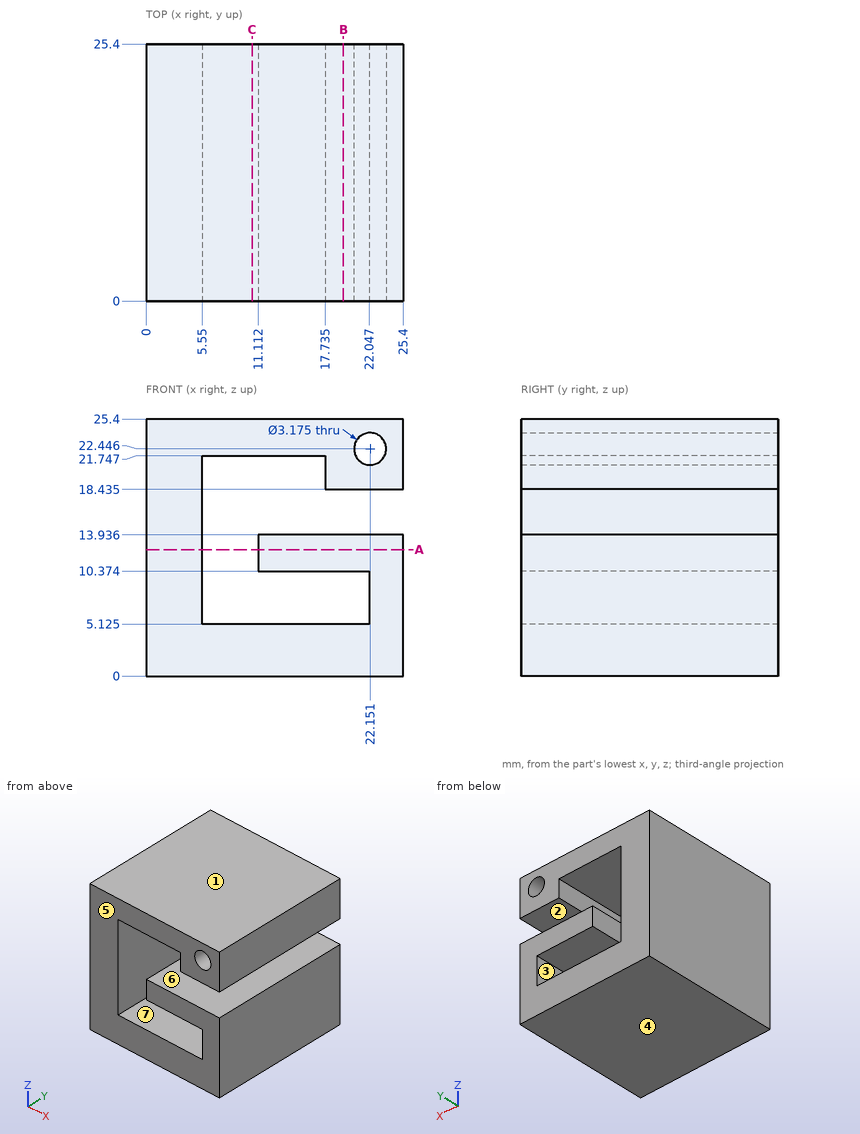
Source: three-view drawing plus pictorial views. Frame: mm from the lowest corner of the part. A direction names the side the tool comes from. Round coordinates to 2 decimals unless told otherwise and drop trailing zeros. Loops run counter-clockwise (first coordinate to the right, second up) from the corner with the lowest first, then second, coordinate; pieces in that order, holes last. Notation, with made-up numbers: (-11.5, 57) -> (28.5, 57) arc R30 ccw to (28.5, 81) -> close; hole circle Ø11 at (-24.75, 4.5). An arc over 180 degrees is marked (long way). Use one line per item in the form item = value.
Item 1: Material intervals for probe 1 along Z at (x, y) = (13, 3.5) (1 decimal); probe 2 along X at (y, z) = (7, 9.5); probe 3 along X at (y, z) = (13, 11.5), sorted ascending.
Evaluation:
probe_1 = 0 to 5.1, 10.4 to 13.9, 21.7 to 25.4
probe_2 = 0 to 5.55, 22.05 to 25.4
probe_3 = 0 to 5.55, 11.11 to 25.4
Item 2: Cut plane B-B on x = 19.5. Output: boundary loops of the cut face in (y, z) (1 decimal).
Evaluation:
outline = (0, 0) -> (25.4, 0) -> (25.4, 5.1) -> (0, 5.1) -> close; (0, 10.4) -> (25.4, 10.4) -> (25.4, 13.9) -> (0, 13.9) -> close; (0, 18.4) -> (25.4, 18.4) -> (25.4, 25.4) -> (0, 25.4) -> close
Item 3: Cut plane A-A on z = 12.5. Output: boundary loops of the cut face in (x, y).
Evaluation:
outline = (0, 0) -> (5.55, 0) -> (5.55, 25.4) -> (0, 25.4) -> close; (11.11, 0) -> (25.4, 0) -> (25.4, 25.4) -> (11.11, 25.4) -> close
Item 4: Access query for the marked faces 5, 6 and 7. Directions: +Z, -Z, +X, -X, +Y, -Y. A direction counts if a zero-diameter tool reaches every point of the face in a straight line with its end or side. Return the directions, or none.
Evaluation:
face_5 = +Z, -Z, +X, -X, -Y
face_6 = +X, +Y, -Y
face_7 = +Y, -Y
Item 5: Cut plane C-C on x = 10.5. Output: boundary loops of the cut face in (y, z) (1 decimal).
Evaluation:
outline = (0, 0) -> (25.4, 0) -> (25.4, 5.1) -> (0, 5.1) -> close; (0, 21.7) -> (25.4, 21.7) -> (25.4, 25.4) -> (0, 25.4) -> close
Item 6: Draft query along Z for the marked faces 1, 2, 3 and 4. Return one class per face: released by +Z, released by -Z, zero draft, split by the parting line, or undercut.
Evaluation:
face_1 = released by +Z
face_2 = undercut
face_3 = undercut
face_4 = released by -Z
